Design review of the part built by this model. Coordinates are the model's own, in mm. Face numbers are marked on the shaded views. A direction names the side the tool comes from. Coordinates: 2 decimals unless noted, no trailing zeros. Write each loop counter-clockwise with the first axis right and the second up, starting at its lowest first coordinate (ties: lowest second). Pieces come first, ordered by that corner, then holes.
Q1. Take a section at B-B, the plane z = 17. Write out the cut boundary in (x, y), plus the area to 4 significant figures.
Q2. For pin 1 Ø1 at (x, z) = (-37.5, -68) entering from +Y; pin 2 Ø3 at (x, z) = (-66.66, -83.03) entering from +Y, all flat-tipped, find the tip position at first contact; note any pin that passes through.
Q3. Take a section at A-A, the plane y = 47.5. Write out the cut boundary in (x, z) (3 decimals), plus the area to 3 significant figures.
Q4. Take a section at C-C, the plane x = -14. Write out the cut boundary in (y, z), plus the area to 3 significant figures.
Q5. For L1, parallel to Z at x = -55, y = 35; L2, parallel to X at y = 27.5, z = -16; L3, parallel to Y at x = -24, z = 2, list the stretches that pass through material, from the lowest coordinate up.
Q6. The part is to be moulded in two halves that separate along X. For the marked faces 1, 2 and 3, say which applies: released by +X, released by -X, zero draft, split by the parting line, or undercut.
Q7. Take a section at D-D, the plane y = 30. Write out the cut boundary in (x, z), plus the area to 3 significant figures.
Q8. For the marked faces 4 and 5, list the 3-axis set-ups (+Z, -Z, +X, -X, +Y, -Y) from which the entire face can be reached by the end or side of a thin tool; tool diameter is ignored.
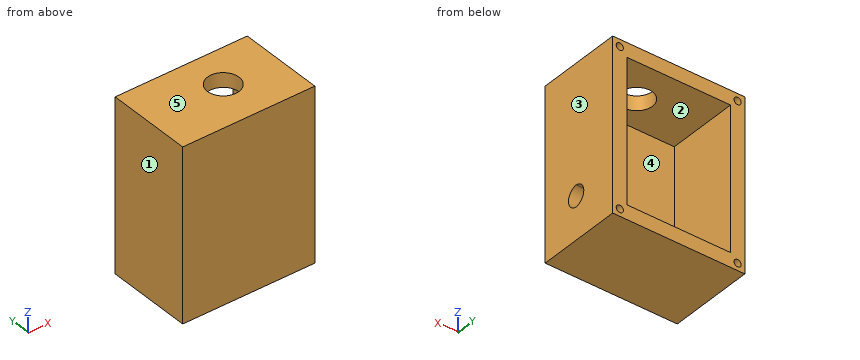
Autodesk Inventor part; units mm, degrees
ref_plane "YZ Plane" through (0, 0, 0) normal (1, 0, 0) x (0, 1, 0)
ref_plane "XZ Plane" through (0, 0, 0) normal (0, 1, 0) x (-1, 0, 0)
ref_plane "XY Plane" through (0, 0, 0) normal (0, 0, 1) x (1, 0, 0)
sketch "Sketch1" plane through (0, 0, 0) normal (0, 1, 0) x (-1, 0, 0)
  line L0 (71.7038, 31.922) -> (71.7038, -88.078)
  line L1 (71.7038, -88.078) -> (-20.7962, -88.078)
  line L2 (-20.7962, -88.078) -> (-20.7962, 31.922)
  line L3 (-20.7962, 31.922) -> (71.7038, 31.922)
  point P0 (0, 0)
  dimension "d0" = 120
  dimension "d1" = 92.5
extrude "Extrusion1" add sketch "Sketch1" along normal blind 60
shell "Shell2" thickness 10 removed faces 1 at (-10.0371, 60, -48.078)
sketch "Sketch12" plane through (0, 60, 0) normal (0, 1, 0) x (1, 0, 0)
  line L0 (10.7962, 78.078) -> (10.7962, -21.922)
  line L1 (10.7962, -21.922) -> (20.7962, -21.922)
  line L2 (20.7962, -31.922) -> (20.7962, 88.078)
  line L3 (20.7962, -21.922) -> (20.7962, -31.922)
  line L4 (20.7962, -31.922) -> (10.7962, -31.922)
  line L5 (10.7962, -31.922) -> (10.7962, -21.922)
  line L6 (20.7962, -31.922) -> (15.8432, -31.922)
  line L7 (-71.7038, -31.922) -> (20.7962, -31.922)
  line L8 (15.8432, -26.969) -> (20.7962, -26.969)
  line L9 (15.8432, -26.969) -> (15.8432, -31.922)
  point P0 (0, 0)
  dimension "d124" = 4.953
  dimension "d125" = 4.953
hole "Hole11" at (15.8432, 60, 26.969) direction (0, -1, 0) diameter 5 depth 25.4 tip angle 118
sketch "Sketch19" plane through (0, 60, 0) normal (0, 1, 0) x (1, 0, 0)
  line L0 (10.7962, -21.922) -> (-61.7038, -21.922)
  line L1 (-61.7038, -21.922) -> (-61.7038, -31.922)
  line L2 (-71.7038, -31.922) -> (20.7962, -31.922)
  line L3 (-71.7038, -31.922) -> (-71.7038, -21.922)
  line L4 (-71.7038, 88.078) -> (-71.7038, -31.922)
  line L5 (-61.7038, -23.8125) -> (-61.7038, -21.922)
  line L6 (-71.7038, -21.922) -> (-61.7038, -21.922)
  line L7 (-61.7038, -21.922) -> (-61.7038, 78.078)
  line L8 (-61.7038, -21.922) -> (-66.7038, -21.922)
  line L9 (-66.6566, -26.875) -> (-61.7038, -26.922)
  line L10 (-66.6566, -26.875) -> (-66.7038, -21.922)
  point P0 (0, 0)
  dimension "d133" = 4.953
  dimension "d134" = 4.953
hole "Hole12" at (-66.6566, 60, 26.875) direction (0, -1, 0) diameter 5 depth 25.4 tip angle 118
sketch "Sketch21" plane through (0, 60, 0) normal (0, 1, 0) x (1, 0, 0)
  line L0 (10.7962, -21.922) -> (10.7962, 78.078)
  line L1 (10.7962, 78.078) -> (20.7962, 78.078)
  line L2 (20.7962, -31.922) -> (20.7962, 88.078)
  line L3 (20.7962, 88.078) -> (10.7962, 88.078)
  line L4 (20.7962, 88.078) -> (-71.7038, 88.078)
  line L5 (10.7962, 78.078) -> (10.7962, 88.078)
  line L6 (10.7962, 78.078) -> (-61.7038, 78.078)
  line L7 (10.7962, 78.078) -> (15.7962, 78.078)
  line L8 (15.8432, 83.031) -> (20.7962, 83.031)
  line L9 (15.8432, 83.031) -> (15.7962, 78.078)
  point P0 (0, 0)
  dimension "d146" = 4.953
hole "Hole13" at (15.8432, 60, -83.031) direction (0, -1, 0) diameter 5 depth 25.4 tip angle 118
sketch "Sketch22" plane through (0, 60, 0) normal (0, 1, 0) x (1, 0, 0)
  line L0 (-61.7038, 78.078) -> (10.7962, 78.078)
  line L1 (-61.7038, 78.078) -> (-71.7038, 78.078)
  line L2 (-71.7038, 88.078) -> (-71.7038, -31.922)
  line L3 (-71.7038, 88.078) -> (-61.7038, 88.078)
  line L4 (20.7962, 88.078) -> (-71.7038, 88.078)
  line L5 (-61.7038, 78.078) -> (-61.7038, 88.078)
  line L6 (-61.7038, 78.078) -> (-66.7038, 78.078)
  line L7 (-66.6568, 83.031) -> (-61.7038, 83.031)
  line L8 (-66.6568, 83.031) -> (-66.7038, 78.078)
  point P0 (0, 0)
  dimension "d155" = 4.953
  dimension "d156" = 4.953
hole "Hole14" at (-66.6568, 60, -83.031) direction (0, -1, 0) diameter 5 depth 25.4 tip angle 118
sketch "Sketch23" plane through (-71.7038, 0, 31.922) normal (0, 0, 1) x (1, 0, 0)
  point P0 (71.7038, 0)
sketch "Sketch24" plane through (-71.7038, 0, 31.922) normal (0, 0, 1) x (1, 0, 0)
  line L0 (0, 0) -> (0, 60)
  line L1 (0, 60) -> (0, 0)
  line L2 (0, 0) -> (92.5, 0)
  line L3 (0, 0) -> (92.5, 0)
  line L4 (92.5, 0) -> (92.5, 60)
  line L5 (92.5, 0) -> (92.5, 60)
  line L6 (0, 60) -> (92.5, 60)
  line L7 (92.5, 60) -> (0, 60)
  line L8 (0, 32.5045) -> (54, 32.5045)
  line L9 (54, 32.5045) -> (46.25, 60)
  line L10 (82.5, 60) -> (10, 60)
  point P0 (71.7038, 0)
  dimension "d164" = 60
  dimension "d165" = 92.5
  dimension "d175" = 54
  dimension "d176" = 27.4955
hole "Hole15" at (-17.7038, 32.5045, 31.922) direction (0, 0, -1) diameter 22 depth 25.4 tip angle 118
sketch "Sketch32" plane through (20.7962, 0, 31.922) normal (1, 0, 0) x (0, 0, -1)
  line L0 (0, 60) -> (120, 60)
  line L1 (90, 60) -> (90, 32.5)
  line L2 (90, 32.5) -> (120, 32.5)
  line L3 (120, 0) -> (120, 60)
  point P0 (31.922, 0)
  dimension "d189" = 27.5
  dimension "d190" = 30
sketch "Sketch33" plane through (20.7962, 0, 31.922) normal (1, 0, 0) x (0, 0, -1)
  line L0 (89.9856, 20.7094) -> (89.9856, 34.3094) construction
  line L1 (82.4856, 28.2094) -> (82.4856, 26.8094)
  line L2 (97.4856, 26.8094) -> (97.4856, 28.2094)
  arc A0 (82.4856, 28.2094) -> (97.4856, 28.2094) centre (89.9856, 28.2094) ccw
  arc A1 (97.4856, 26.8094) -> (82.4856, 26.8094) centre (89.9856, 26.8094) ccw
  point P0 (31.922, 0)
  point P1 (89.9856, 27.5094)
  point P2 (97.4528, 27.5094)
  point P3 (82.5183, 27.5094)
  dimension "d191" = 13.6
  dimension "d192" = 7.5
extrude "Extrusion2" cut sketch "Sketch33" against normal blind 10 contours A1 A0
sketch "Sketch35" plane through (-71.7038, 0, 31.922) normal (0, 0, 1) x (1, 0, 0)
  circle A0 centre (54, 32.5045) radius 11
  line L0 (43, 32.5045) -> (-0.012, 32.5045)
  line L1 (10, 10) -> (10, 60)
  point P0 (71.7038, 0)
  dimension "d195" = 43.012
properties part number "Water_Proof_Box_Bottom"
Responses:
1. outline: (-71.7, 0) - (20.8, 0) - (20.8, 60) - (10.8, 60) - (10.8, 10) - (-61.7, 10) - (-61.7, 60) - (-71.7, 60) - close
1. area: 1,925 mm2
2. pin 1: stops at y = 10
2. pin 2: stops at y = 34
3. outline: (-71.704, -88.078) - (20.796, -88.078) - (20.796, 31.922) - (-71.704, 31.922) - close; hole circle Ø5 at (-66.657, -83.031); hole circle Ø5 at (-66.657, 26.875); hole (-61.704, -78.078) - (10.796, -78.078) - (10.796, 21.922) - (-61.704, 21.922) - close; hole circle Ø5 at (15.843, -83.031); hole circle Ø5 at (15.843, 26.969)
3. area: 3,770 mm2
4. outline: (0, -88.08) - (60, -88.08) - (60, -78.08) - (10, -78.08) - (10, 21.92) - (22.15, 21.92) - (22.15, 31.92) - (0, 31.92) - close; (42.86, 21.92) - (60, 21.92) - (60, 31.92) - (42.86, 31.92) - close
4. area: 1,990 mm2
5. L1: z = -88.08 to -78.08, 21.92 to 31.92
5. L2: x = -71.7 to -61.7, 10.8 to 20.8
5. L3: y = 0 to 10
6. face 1: released by -X
6. face 2: undercut
6. face 3: released by +X
7. outline: (-71.7, -88.08) - (20.8, -88.08) - (20.8, -64.85) - (10.8, -64.85) - (10.8, -78.08) - (-61.7, -78.08) - (-61.7, 21.92) - (-28.41, 21.92) - (-28.41, 31.92) - (-71.7, 31.92) - close; (-6.99, 21.92) - (10.8, 21.92) - (10.8, -51.28) - (20.8, -51.28) - (20.8, 31.92) - (-6.99, 31.92) - close
7. area: 3,500 mm2
8. face 4: +Y
8. face 5: +Z, +X, -X, +Y, -Y
